Geometry check sheet. Reference: the model listing, model coordinates, mm. Face numbers are marked on the shaded views. A direction names the side the tool comes from. Round coordinates to 2 decimals unless told otherwise and drop trailing zeros. Write each loop counter-clockwise with the first axis right and the second up, starting at its lowest first coordinate (ties: lowest second). Pieces come first, ordered by that corner, then holes. Notation, with made-up numbers: (-39.75, -30) -> (14.25, -30) arc R12 ccw to (14.25, -24) -> close; hole circle Ø7 at (60, -20). An arc over 180 degrees is marked (long way). Use a Markdown table: item, result.
Autodesk Inventor part; units mm, degrees
ref_plane "YZ Plane" through (0, 0, 0) normal (1, 0, 0) x (0, 1, 0)
ref_plane "XZ Plane" through (0, 0, 0) normal (0, 1, 0) x (-1, 0, 0)
ref_plane "XY Plane" through (0, 0, 0) normal (0, 0, 1) x (1, 0, 0)
sketch "Sketch1" plane through (0, 0, 0) normal (0, 0, 1) x (1, 0, 0)
  line L0 (0, 0) -> (12, 0)
  line L1 (13, 1) -> (13, 18.7)
  line L2 (14, 19.7) -> (51, 19.7)
  line L3 (52, 18.7) -> (52, 1)
  line L4 (53, 0) -> (65, 0)
  line L5 (65, 0) -> (65, 3)
  line L6 (65, 3) -> (56, 3)
  line L7 (55, 4) -> (55, 21.7)
  line L8 (54, 22.7) -> (11, 22.7)
  line L9 (10, 21.7) -> (10, 4)
  line L10 (9, 3) -> (0, 3)
  line L11 (0, 3) -> (0, 0)
  arc A0 (11, 22.7) -> (10, 21.7) centre (11, 21.7) ccw
  arc A1 (14, 19.7) -> (13, 18.7) centre (14, 18.7) ccw
  arc A2 (9, 3) -> (10, 4) centre (9, 4) ccw
  arc A3 (12, 0) -> (13, 1) centre (12, 1) ccw
  arc A4 (55, 4) -> (56, 3) centre (56, 4) ccw
  arc A5 (55, 21.7) -> (54, 22.7) centre (54, 21.7) ccw
  arc A6 (52, 18.7) -> (51, 19.7) centre (51, 18.7) ccw
  arc A7 (52, 1) -> (53, 0) centre (53, 1) ccw
  point P0 (52, 0)
  dimension "d0" = 3
  dimension "d1" = 3
  dimension "d2" = 3
  dimension "d3" = 3
  dimension "d4" = 3
  dimension "d5" = 19.7
  dimension "d6" = 39
  dimension "d7" = 10
  dimension "d8" = 10
  dimension "d9" = 1
  dimension "d10" = 1
extrude "Extrusion1" add sketch "Sketch1" along normal blind 15
sketch "Sketch2" plane through (0, 3, 0) normal (0, 1, 0) x (1, 0, 0)
  line L0 (65, 0) -> (56, 0)
  line L1 (65, -15) -> (56, -15)
  line L2 (9, 0) -> (0, 0)
  line L3 (9, -15) -> (0, -15)
  line L4 (65, 0) -> (65, -15)
  line L5 (0, 0) -> (0, -15)
  point P0 (60, -4)
  point P1 (60, -11)
  point P2 (5, -11)
  point P3 (5, -4)
  dimension "d13" = 4
  dimension "d14" = 4
  dimension "d15" = 4
  dimension "d16" = 4
  dimension "d17" = 5
  dimension "d18" = 5
  dimension "d19" = 5
  dimension "d20" = 5
hole "Hole1" at (60, 3, 4) at (60, 3, 11) at (5, 3, 11) at (5, 3, 4) direction (0, -1, 0) diameter 3.4 end through all
properties part number "servoPlateConnection"
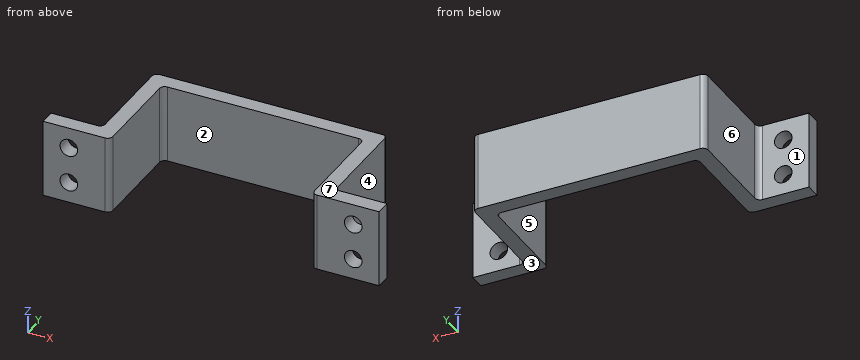
(1) Section check C-C on y = 5.75. Record the cut outline in (x, z), plus the area to 3 significant figures.
A:
| item | result |
|---|---|
| outline | (10, 0) -> (13, 0) -> (13, 15) -> (10, 15) -> close; (52, 0) -> (55, 0) -> (55, 15) -> (52, 15) -> close |
| area | 90.0 mm2 |
(2) Release check for a two-part mould opening along X. For the marked faces 5, 6 and 7 record: +X half, -X half, draft (parallel to the pull), parting line (faces both ways), or undercut.
A:
| item | result |
|---|---|
| face 5 | undercut |
| face 6 | -X half |
| face 7 | draft |
(3) Thickness scan on line 1 (Z direction, x = 60, y = 0.8); line 2 (X direction, y = 2.2, z = 11); line 3 (X direction, y = 13.25, z = 5.5). Record the ranges inside material, lowest first.
A:
| item | result |
|---|---|
| line 1 | z = 0 to 2.3, 5.7 to 9.3, 12.7 to 15 |
| line 2 | x = 0 to 3.3, 6.7 to 13, 52 to 58.3, 61.7 to 65 |
| line 3 | x = 10 to 13, 52 to 55 |
(4) Section check D-D on y = 20.5. Record the cut outline in (x, z).
A:
| item | result |
|---|---|
| outline | (10, 0) -> (55, 0) -> (55, 15) -> (10, 15) -> close |
(5) Section check A-A on z = 4. Record the cut outline in (x, y), plus the area to 3 significant figures.
A:
| item | result |
|---|---|
| outline | (0, 0) -> (3.3, 0) -> (3.3, 3) -> (0, 3) -> close; (6.7, 0) -> (12, 0) arc R1 ccw to (13, 1) -> (13, 18.7) arc R1 cw to (14, 19.7) -> (51, 19.7) arc R1 cw to (52, 18.7) -> (52, 1) arc R1 ccw to (53, 0) -> (58.3, 0) -> (58.3, 3) -> (56, 3) arc R1 cw to (55, 4) -> (55, 21.7) arc R1 ccw to (54, 22.7) -> (11, 22.7) arc R1 ccw to (10, 21.7) -> (10, 4) arc R1 cw to (9, 3) -> (6.7, 3) -> close; (61.7, 0) -> (65, 0) -> (65, 3) -> (61.7, 3) -> close |
| area | 293 mm2 |
(6) Access from +Z, -Z, +X, -X, +Y, -Y to the whole of each face (thin tool, end or side, straight path). Record for the marked faces 1, 2, 3 and 4.
A:
| item | result |
|---|---|
| face 1 | +Z, -Z, -X, +Y |
| face 2 | +Z, -Z, -Y |
| face 3 | -Z, +X, -X, +Y, -Y |
| face 4 | +Z, -Z, +X, +Y |
(7) Section check B-B on x = 5. Record the cut outline in (y, z), plus the area to 3 significant figures.
A:
| item | result |
|---|---|
| outline | (0, 0) -> (3, 0) -> (3, 2.3) -> (0, 2.3) -> close; (0, 5.7) -> (3, 5.7) -> (3, 9.3) -> (0, 9.3) -> close; (0, 12.7) -> (3, 12.7) -> (3, 15) -> (0, 15) -> close |
| area | 24.6 mm2 |
(8) Gauge pin test, flat ends, axial feed: pin 1 Ø4.5 at (y, z) = (17, 8.5) entering from -X; pin 2 Ø2 at (x, y) = (55.5, 16.5) entering from +Z; pin 3 Ø4.5 at (y, z) = (16.5, 11) entering from +X; pin 4 Ø3 at (x, z) = (5, 11) entering from -Y. Record the tip position at first contact, or that the pin passes through.
A:
| item | result |
|---|---|
| pin 1 | stops at x = 10 |
| pin 2 | stops at z = 15 |
| pin 3 | stops at x = 55 |
| pin 4 | passes through |
